from build123d import *

# Parameters (mm, degrees)
SKETCH_1_R          = 13.5
SKETCH_1_R_2        = 1.6
SKETCH_1_R_3        = 2.1
SKETCH_1_R_4        = 1.35
SKETCH_1_R_5        = 1.5
EXTRUDE_1_DEPTH     = 5
FILLET_1_R          = 10
FILLET_2_R          = 4
FILLET_3_R          = 2
CUT_EXTRUDE_1_DEPTH = 109.282039139
SKETCH_3_W          = 26
SKETCH_3_H          = 20
CUT_EXTRUDE_2_DEPTH = 109.282039139


with BuildPart() as part:
    # 草图1 → 凸台-拉伸1 (new body)
    with BuildSketch(Plane.XY):
        with BuildLine():
            Line((-42.5, -55.5), (-30, -55.5))
            Line((-30, -55.5), (-30, -87.5))
            Line((-30, -87.5), (-20, -87.5))
            Line((-20, -87.5), (-20, -55.5))
            Line((-20, -55.5), (20, -55.5))
            Line((20, -55.5), (20, -87.5))
            Line((20, -87.5), (30, -87.5))
            Line((30, -87.5), (30, -55.5))
            Line((30, -55.5), (42.5, -55.5))
            Line((42.5, -55.5), (60, -25.189110868))
            Line((60, -25.189110868), (60, -13.189110868))
            Line((60, -13.189110868), (43, 0.5))
            Line((43, 0.5), (31, 0.5))
            Line((31, 0.5), (31, 88))
            ThreePointArc((31, 88), (30.414213562, 89.414213562), (29, 90))
            Line((29, 90), (-29, 90))
            ThreePointArc((-29, 90), (-30.414213562, 89.414213562), (-31, 88))
            Line((-31, 88), (-31, 0.5))
            Line((-31, 0.5), (-43, 0.5))
            Line((-43, 0.5), (-60, -13.189110868))
            Line((-60, -13.189110868), (-60, -25.189110868))
            Line((-60, -25.189110868), (-42.5, -55.5))
        make_face()
        with Locations((36.5, -24)):
            Circle(SKETCH_1_R, mode=Mode.SUBTRACT)
        with Locations((32.902497054, -6.87376362)):
            Circle(SKETCH_1_R_2, mode=Mode.SUBTRACT)
        with Locations((53.62623638, -20.402497054)):
            Circle(SKETCH_1_R_2, mode=Mode.SUBTRACT)
        with Locations((19.37376362, -27.597502946)):
            Circle(SKETCH_1_R_2, mode=Mode.SUBTRACT)
        with Locations((40.097502946, -41.12623638)):
            Circle(SKETCH_1_R_2, mode=Mode.SUBTRACT)
        with Locations((-36.5, -24)):
            Circle(SKETCH_1_R, mode=Mode.SUBTRACT)
        with Locations((-40.097502946, -6.87376362)):
            Circle(SKETCH_1_R_2, mode=Mode.SUBTRACT)
        with Locations((-19.37376362, -20.402497054)):
            Circle(SKETCH_1_R_2, mode=Mode.SUBTRACT)
        with Locations((-32.902497054, -41.12623638)):
            Circle(SKETCH_1_R_2, mode=Mode.SUBTRACT)
        with Locations((-53.62623638, -27.597502946)):
            Circle(SKETCH_1_R_2, mode=Mode.SUBTRACT)
        with Locations((-13, -51.5)):
            Circle(SKETCH_1_R_3, mode=Mode.SUBTRACT)
        with Locations((13, -51.5)):
            Circle(SKETCH_1_R_3, mode=Mode.SUBTRACT)
        with Locations((0, -24)):
            Circle(SKETCH_1_R_3, mode=Mode.SUBTRACT)
        with Locations((27, 21)):
            Circle(SKETCH_1_R_3, mode=Mode.SUBTRACT)
        with Locations((27, 61)):
            Circle(SKETCH_1_R_3, mode=Mode.SUBTRACT)
        with Locations(Location((-27, 21, 0), (0, 0, 180))):
            Circle(SKETCH_1_R_3, mode=Mode.SUBTRACT)
        with Locations(Location((-27, 61, 0), (0, 0, 180))):
            Circle(SKETCH_1_R_3, mode=Mode.SUBTRACT)
        with Locations((-25, -79.5)):
            Circle(SKETCH_1_R_2, mode=Mode.SUBTRACT)
        with Locations((-25, -63.5)):
            Circle(SKETCH_1_R_2, mode=Mode.SUBTRACT)
        with Locations((-25, -71.5)):
            Circle(SKETCH_1_R_2, mode=Mode.SUBTRACT)
        with Locations(Location((25, -79.5, 0), (0, 0, 180))):
            Circle(SKETCH_1_R_2, mode=Mode.SUBTRACT)
        with Locations(Location((25, -71.5, 0), (0, 0, 180))):
            Circle(SKETCH_1_R_2, mode=Mode.SUBTRACT)
        with Locations(Location((25, -63.5, 0), (0, 0, 180))):
            Circle(SKETCH_1_R_2, mode=Mode.SUBTRACT)
        with Locations((14, 23.5)):
            Circle(SKETCH_1_R_4, mode=Mode.SUBTRACT)
        with Locations((-14, 23.5)):
            Circle(SKETCH_1_R_4, mode=Mode.SUBTRACT)
        with Locations((14, 66.5)):
            Circle(SKETCH_1_R_4, mode=Mode.SUBTRACT)
        with Locations((-14, 66.5)):
            Circle(SKETCH_1_R_4, mode=Mode.SUBTRACT)
        with Locations((-23, 83)):
            Circle(SKETCH_1_R_2, mode=Mode.SUBTRACT)
        with Locations((23, 83)):
            Circle(SKETCH_1_R_2, mode=Mode.SUBTRACT)
        with Locations((23, 1.5)):
            Circle(SKETCH_1_R_5, mode=Mode.SUBTRACT)
        with Locations((-23, 1.5)):
            Circle(SKETCH_1_R_5, mode=Mode.SUBTRACT)
    extrude(amount=EXTRUDE_1_DEPTH)

    # 圆角1
    fillet_1_edges = [part.edges().sort_by_distance(p)[0] for p in [
        (-42.5, -55.5, 2.5),
        (-60, -25.189110868, 2.5),
        (-60, -13.189110868, 2.5),
        (-43, 0.5, 2.5),
        (43, 0.5, 2.5),
        (60, -13.189110868, 2.5),
        (60, -25.189110868, 2.5),
        (42.5, -55.5, 2.5),
    ]]
    fillet(fillet_1_edges, radius=FILLET_1_R)

    # 圆角2
    fillet_2_edges = [part.edges().sort_by_distance(p)[0] for p in [
        (-31, 0.5, 2.5),
        (31, 0.5, 2.5),
    ]]
    fillet(fillet_2_edges, radius=FILLET_2_R)

    # 圆角3
    fillet_3_edges = [part.edges().sort_by_distance(p)[0] for p in [
        (30, -55.5, 2.5),
        (30, -87.5, 2.5),
        (20, -87.5, 2.5),
        (20, -55.5, 2.5),
        (-20, -55.5, 2.5),
        (-20, -87.5, 2.5),
        (-30, -87.5, 2.5),
        (-30, -55.5, 2.5),
    ]]
    fillet(fillet_3_edges, radius=FILLET_3_R)

    # 草图2 → 切除-拉伸1 (cut, through all)
    with BuildSketch(Plane.XY.offset(5)):
        with BuildLine():
            Line((10.051800354, -18.412507883), (0.948199646, -13.51056904))
            ThreePointArc((0.948199646, -13.51056904), (0, -13.27151124), (-0.948199646, -13.51056904))
            Line((-0.948199646, -13.51056904), (-10.051800354, -18.412507883))
            ThreePointArc((-10.051800354, -18.412507883), (-12.025573183, -18.368597903), (-13, -16.651565683))
            Line((-13, -16.651565683), (-13, -2))
            ThreePointArc((-13, -2), (-12.414213562, -0.585786438), (-11, 0))
            Line((-11, 0), (11, 0))
            ThreePointArc((11, 0), (12.414213562, -0.585786438), (13, -2))
            Line((13, -2), (13, -16.651565683))
            ThreePointArc((13, -16.651565683), (12.025573183, -18.368597903), (10.051800354, -18.412507883))
        make_face()
        with BuildLine():
            Line((-8, -35), (-8, -43))
            ThreePointArc((-8, -43), (-7.414213562, -44.414213562), (-6, -45))
            Line((-6, -45), (6, -45))
            ThreePointArc((6, -45), (7.414213562, -44.414213562), (8, -43))
            Line((8, -43), (8, -35))
            ThreePointArc((8, -35), (7.414213562, -33.585786438), (6, -33))
            Line((6, -33), (-6, -33))
            ThreePointArc((-6, -33), (-7.414213562, -33.585786438), (-8, -35))
        make_face()
        with BuildLine():
            Line((-16, 59), (16, 59))
            ThreePointArc((16, 59), (17.414213562, 58.414213562), (18, 57))
            Line((18, 57), (18, 33))
            ThreePointArc((18, 33), (17.414213562, 31.585786438), (16, 31))
            Line((16, 31), (-16, 31))
            ThreePointArc((-16, 31), (-17.414213562, 31.585786438), (-18, 33))
            Line((-18, 33), (-18, 57))
            ThreePointArc((-18, 57), (-17.414213562, 58.414213562), (-16, 59))
        make_face()
        with BuildLine():
            Line((-12, 84), (12, 84))
            ThreePointArc((12, 84), (16, 80), (12, 76))
            Line((12, 76), (-12, 76))
            ThreePointArc((-12, 76), (-16, 80), (-12, 84))
        make_face()
    extrude(amount=-CUT_EXTRUDE_1_DEPTH, mode=Mode.SUBTRACT)

    # 草图3 → 切除-拉伸2 (cut, through all)
    with BuildSketch(Plane.XY.offset(5)):
        with Locations((0, 8)):
            Rectangle(SKETCH_3_W, SKETCH_3_H)
    extrude(amount=-CUT_EXTRUDE_2_DEPTH, mode=Mode.SUBTRACT)


solid = part.part
Model file for the job. Use its own axes, mm. A direction names the side the tool comes from. Give positions to 0.01 mm unless a question says otherwise; leave off trailing zeros. Loops run counter-clockwise (first coordinate to the right, second up) from the corner with the lowest first, then second, coordinate; pieces in that order, holes last. Notation, with made-up numbers: (65, 71.5) -> (114, 71.5) arc R22 ccw to (114, 97.5) -> close; hole circle Ø2 at (-37.5, -16.5). An arc over 180 degrees is marked (long way). Use a Markdown table: item, result. Add a question column.
(1) Slice it at C-C on z = 3.15. Give the number of separate pieces and of enclosed holes in the cut face, and give its area (3 significant figures).
(2) Wall check: line 1 along X through (y, z) = (-79.5, 3.45); line 2 along Y through (x, z) = (37.5, 4.3); line 3 along X through (y, z) = (-8, 2.05). Give the ranges that are in metal, low to high.
(3) Slice it at A-A on y = 10.5. List the corners of the cut face in (x, z).
(4) Slice it at B-B on y = 36. List the corners of the cut face in (x, z).
(5) Tool access for faces 1 (the flat face through (5.564, -15.996, 2.535)), 2 (the flat face through (30, -72, 2)), 3 (the flat face through (-14, 2, 0)), 4 (the flat face through (-37, 0.5, 2)): list every direction of +Z, -Z, +X, -X, +Y, -Y with a clear straight run to the whole face (end or side of a thin tool).
(6) Mould opens along X. For faces 5 (the flat face through (-25, -87.5, 2)), 6 (the flat face through (18, 45, 3)), 7 (the flat face through (-18, 45, 3)), 8 (the flat face through (-50.935, -5.89, 2.465)) say: +X half, -X half, draft (parallel to the pull), parting line (faces both ways), or undercut.
(7) Drop flat-ended pins along their axis: pin 1 Ø1.6 at (x, y) = (14, 66.5) entering from +Z; pin 2 Ø3 at (x, z) = (39.5, 4) entering from -Y. Give the stop position or say it passes through.
Filled sheet:
| question | item | result |
|---|---|---|
| 1 | separate pieces | 1 |
| 1 | enclosed holes | 35 |
| 1 | area | 8,390 mm2 |
| 2 | line 1 | -30 to -26.6, -23.4 to -20, 20 to 23.4, 26.6 to 30 |
| 2 | line 2 | -55.47 to -37.46, -10.54 to 0.5 |
| 2 | line 3 | -53.56 to -41.23, -38.96 to -13, 13 to 31.77, 34.04 to 53.56 |
| 3 | outline | (-31, 0) -> (-13, 0) -> (-13, 5) -> (-31, 5) -> close; (13, 0) -> (31, 0) -> (31, 5) -> (13, 5) -> close |
| 4 | outline | (-31, 0) -> (-18, 0) -> (-18, 5) -> (-31, 5) -> close; (18, 0) -> (31, 0) -> (31, 5) -> (18, 5) -> close |
| 5 | face 1 | +Z, -Z |
| 5 | face 2 | +Z, -Z, +X, -Y |
| 5 | face 3 | -Z, +X, -X, +Y, -Y |
| 5 | face 4 | +Z, -Z, -X, +Y |
| 6 | face 5 | draft |
| 6 | face 6 | undercut |
| 6 | face 7 | undercut |
| 6 | face 8 | -X half |
| 7 | pin 1 | through |
| 7 | pin 2 | y = -55.42 |
